Here's how the part is built. I have some questions about the finished solid (model axes, mm). A direction names the side the tool comes from. Round coordinates to 2 decimals unless told otherwise and drop trailing zeros. Loops run counter-clockwise (first coordinate to the right, second up) from the corner with the lowest first, then second, coordinate; pieces in that order, holes last. Notation, with made-up numbers: (59, -9) -> (95, -9) arc R22 cw to (95, -3) -> close; hole circle Ø8 at (60, 60). An arc over 180 degrees is marked (long way). One line per item, written item: value. Start each with the question number.
```python
from build123d import *

# Parameters (mm, degrees)
AUFSATZ_LINEAR_AUSTRAGEN1_OUTLINE_W = 29
AUFSATZ_LINEAR_AUSTRAGEN1_OUTLINE_H = 29
AUFSATZ_LINEAR_AUSTRAGEN1_DEPTH     = 2
SKIZZE2_W                           = 19
SKIZZE2_H                           = 24
AUFSATZ_LINEAR_AUSTRAGEN2_DEPTH     = 18
SKIZZE5_W                           = 15
SKIZZE5_H                           = 24
SCHNITT_LINEAR_AUSTRAGEN2_DEPTH     = 15
SCHNITT_LINEAR_AUSTRAGEN3_REACH     = 44.626
SKIZZE4_R                           = 1.25
SKIZZE6_W                           = 35
SKIZZE6_H                           = 24
AUFSATZ_LINEAR_AUSTRAGEN3_DEPTH     = 7
SKIZZE9_R                           = 2
SCHNITT_LINEAR_AUSTRAGEN4_DEPTH     = 5
SKIZZE19_W                          = 17
SKIZZE19_H                          = 5
SCHNITT_LINEAR_AUSTRAGEN15_DEPTH    = 2
SKIZZE20_R                          = 1.5
SCHNITT_LINEAR_AUSTRAGEN16_DEPTH    = 2
SKIZZE21_W                          = 7
SKIZZE21_H                          = 8
SCHNITT_LINEAR_AUSTRAGEN17_DEPTH    = 2
SKIZZE23_W                          = 6.5
SKIZZE23_H                          = 5
SKIZZE23_W_2                        = 5.5
SCHNITT_LINEAR_AUSTRAGEN18_DEPTH    = 2
SKIZZE24_W                          = 29
SKIZZE24_H                          = 2
AUFSATZ_LINEAR_AUSTRAGEN4_DEPTH     = 5
SKIZZE25_R                          = 1
SCHNITT_LINEAR_AUSTRAGEN19_DEPTH    = 2
SKIZZE26_W                          = 35
SKIZZE26_H                          = 3
SCHNITT_LINEAR_AUSTRAGEN20_DEPTH    = 7
SKIZZE27_R                          = 3.5
SCHNITT_LINEAR_AUSTRAGEN21_DEPTH    = 2


# Read off the part's stored shape, not the designer's step: Aufsatz-Linear austragen1
with BuildPart() as part:
    # Aufsatz-Linear austragen1 outline → Aufsatz-Linear austragen1 (new body)
    with BuildSketch(Plane.XY):
        with Locations((14.5, 14.5)):
            Rectangle(AUFSATZ_LINEAR_AUSTRAGEN1_OUTLINE_W, AUFSATZ_LINEAR_AUSTRAGEN1_OUTLINE_H)
    extrude(amount=AUFSATZ_LINEAR_AUSTRAGEN1_DEPTH)

    # Skizze2 → Aufsatz-Linear austragen2 (add)
    with BuildSketch(Plane.XY.offset(2)):
        with Locations((14.5, 17)):
            Rectangle(SKIZZE2_W, SKIZZE2_H)
    extrude(amount=AUFSATZ_LINEAR_AUSTRAGEN2_DEPTH)

    # Skizze5 → Schnitt-Linear austragen2 (cut)
    with BuildSketch(Plane.XY.offset(20)):
        with Locations((14.5, 17)):
            Rectangle(SKIZZE5_W, SKIZZE5_H)
    extrude(amount=-SCHNITT_LINEAR_AUSTRAGEN2_DEPTH, mode=Mode.SUBTRACT)

    # Schnitt-Linear austragen3: up to this face of the body (flat: up to its plane)
    schnitt_linear_austragen3_end = Plane(part.part.faces().sort_by_distance((24, 17, 11))[0])
    # Skizze4 → Schnitt-Linear austragen3 (cut, up to the picked face)
    with BuildSketch(Plane.ZY.offset(-5), mode=Mode.PRIVATE) as schnitt_linear_austragen3_sk1:
        with Locations((12, 15)):
            Circle(SKIZZE4_R)
    schnitt_linear_austragen3_tool1 = split(extrude(schnitt_linear_austragen3_sk1.sketch, amount=-SCHNITT_LINEAR_AUSTRAGEN3_REACH, mode=Mode.PRIVATE), bisect_by=schnitt_linear_austragen3_end, keep=Keep.BOTH, mode=Mode.PRIVATE)
    add(schnitt_linear_austragen3_tool1.solids().sort_by(Axis((5, 15, 12), (1, 0, 0)))[0], mode=Mode.SUBTRACT)

    # Skizze6 → Aufsatz-Linear austragen3 (add)
    with BuildSketch(Plane.XY.offset(20)):
        with Locations((14.5, 17)):
            Rectangle(SKIZZE6_W, SKIZZE6_H)
    extrude(amount=AUFSATZ_LINEAR_AUSTRAGEN3_DEPTH)

    # Skizze9 → Schnitt-Linear austragen4 (cut)
    with BuildSketch(Plane(origin=(0, 0, 20), x_dir=(-1, 0, 0), z_dir=(0, 0, -1))):
        with Locations((-1.5, 14)):
            Circle(SKIZZE9_R)
        with Locations((-27.5, 14)):
            Circle(SKIZZE9_R)
    extrude(amount=-SCHNITT_LINEAR_AUSTRAGEN4_DEPTH, mode=Mode.SUBTRACT)

    # Skizze19 → Schnitt-Linear austragen15 (cut)
    with BuildSketch(Plane(origin=(0, 0, 0), x_dir=(-1, 0, 0), z_dir=(0, 0, -1))):
        with Locations((-14, 2.5)):
            Rectangle(SKIZZE19_W, SKIZZE19_H)
    extrude(amount=-SCHNITT_LINEAR_AUSTRAGEN15_DEPTH, mode=Mode.SUBTRACT)

    # Skizze20 → Schnitt-Linear austragen16 (cut)
    with BuildSketch(Plane(origin=(0, 0, 25), x_dir=(-1, 0, 0), z_dir=(0, 0, -1))):
        with Locations((-27.5, 14)):
            Circle(SKIZZE20_R)
        with Locations((-1.5, 14)):
            Circle(SKIZZE20_R)
    extrude(amount=-SCHNITT_LINEAR_AUSTRAGEN16_DEPTH, mode=Mode.SUBTRACT)

    # Skizze21 → Schnitt-Linear austragen17 (cut)
    with BuildSketch(Plane.XY.offset(5)):
        with Locations((14.5, 25)):
            Rectangle(SKIZZE21_W, SKIZZE21_H)
    extrude(amount=-SCHNITT_LINEAR_AUSTRAGEN17_DEPTH, mode=Mode.SUBTRACT)

    # Skizze23 → Schnitt-Linear austragen18 (cut)
    with BuildSketch(Plane(origin=(0, 0, 0), x_dir=(-1, 0, 0), z_dir=(0, 0, -1))):
        with Locations((-25.75, 2.5)):
            Rectangle(SKIZZE23_W, SKIZZE23_H)
        with Locations((-2.75, 2.5)):
            Rectangle(SKIZZE23_W_2, SKIZZE23_H)
    extrude(amount=-SCHNITT_LINEAR_AUSTRAGEN18_DEPTH, mode=Mode.SUBTRACT)

    # Skizze24 → Aufsatz-Linear austragen4 (add)
    with BuildSketch(Plane(origin=(0, 29, 0), x_dir=(1, 0, 0), z_dir=(0, 1, 0))):
        with Locations((14.5, -1)):
            Rectangle(SKIZZE24_W, SKIZZE24_H)
    extrude(amount=AUFSATZ_LINEAR_AUSTRAGEN4_DEPTH)

    # Skizze25 → Schnitt-Linear austragen19 (cut)
    with BuildSketch(Plane(origin=(0, 0, 0), x_dir=(-1, 0, 0), z_dir=(0, 0, -1))):
        with Locations((-1.75, 32.25)):
            Circle(SKIZZE25_R)
        with Locations((-27.25, 32.25)):
            Circle(SKIZZE25_R)
        with Locations((-27.25, 6.75)):
            Circle(SKIZZE25_R)
        with Locations((-1.75, 6.75)):
            Circle(SKIZZE25_R)
    extrude(amount=-SCHNITT_LINEAR_AUSTRAGEN19_DEPTH, mode=Mode.SUBTRACT)

    # Skizze26 → Schnitt-Linear austragen20 (cut)
    with BuildSketch(Plane.XY.offset(27)):
        with Locations((14.5, 27.5)):
            Rectangle(SKIZZE26_W, SKIZZE26_H)
    extrude(amount=-SCHNITT_LINEAR_AUSTRAGEN20_DEPTH, mode=Mode.SUBTRACT)

    # Skizze27 → Schnitt-Linear austragen21 (cut)
    with BuildSketch(Plane(origin=(0, 0, 0), x_dir=(-1, 0, 0), z_dir=(0, 0, -1))):
        with Locations((-27.5, 14)):
            Circle(SKIZZE27_R)
        with Locations((-1.5, 14)):
            Circle(SKIZZE27_R)
    extrude(amount=-SCHNITT_LINEAR_AUSTRAGEN21_DEPTH, mode=Mode.SUBTRACT)


solid = part.part
```
Q1. Will these pins go through, and if not, where does the flat tip stop? P1, Ø0.6, axis at x = 16, z = 4.5, coming from the +Y side; P2, Ø5, axis at y = 14, z = 17, coming from the -X side; P3, Ø1, axis at y = 24.5, z = 4, coming from the +X side.
Q2. If we mould it in two halves opening along Z, with no side actions, what happens to faces 5 (the flat face through (23, 28, 20)), 6 (the flat face through (14, 26, 24)), 7 (the flat face through (11, 31, 2))? For each: released by +Z, released by -Z, zero draft, split by the parting line, or undercut.
Q3. I want a section at A-A on y = 32.25. Please give me the cut outline in (x, z), plus the area to 3 significant figures.
Q4. I want a section at C-C on z = 18.75. Please give me the cut outline in (x, y), plus the area to 3 significant figures.
Q5. I want a section at B-B on x = 12. Please give me the cut outline in (y, z), plus the area to 3 significant figures.
Q6. I want a section at D-D on y = 6.75. Please give me the cut outline in (x, z), plus the area to 3 significant figures.
Q7. If I drill on line 1 along Y through (x, z) = (27.5, 22.3); line 2 along Z through (x, y) = (8, 23.25); line 3 along X through (y, z) = (28.5, 17), over which ranges is the centre line in solid material (lowest first)?
Q8. Which directions (+Z, -Z, +X, -X, +Y, -Y) give clear straight access to the entire face, cutting with the end or side of a thin tool? Please do faces 1 (the flat face through (29, 8, 1)), 2 (the flat face through (18, 25, 4)), 3 (the flat face through (0, 25, 1)), 4 (the cylindrical face through (27.987, 7.426, 0.986)).
Answers below:
1. P1: stops at y = 21
1. P2: stops at x = 5
1. P3: stops at x = 24
2. face 5: released by +Z
2. face 6: zero draft
2. face 7: undercut
3. outline: (0, 0) -> (0.75, 0) -> (0.75, 2) -> (0, 2) -> close; (2.75, 0) -> (26.25, 0) -> (26.25, 2) -> (2.75, 2) -> close; (28.25, 0) -> (29, 0) -> (29, 2) -> (28.25, 2) -> close
3. area: 50.0 mm^2
4. outline: (5, 5) -> (7, 5) -> (7, 29) -> (5, 29) -> close; (22, 5) -> (24, 5) -> (24, 29) -> (22, 29) -> close
4. area: 96.0 mm^2
5. outline: (5, 0) -> (34, 0) -> (34, 2) -> (29, 2) -> (29, 3) -> (21, 3) -> (21, 5) -> (5, 5) -> close; (5, 20) -> (26, 20) -> (26, 27) -> (5, 27) -> close
5. area: 261 mm^2
6. outline: (-3, 20) -> (5, 20) -> (5, 2) -> (2.75, 2) -> (2.75, 0) -> (26.25, 0) -> (26.25, 2) -> (24, 2) -> (24, 20) -> (32, 20) -> (32, 27) -> (-3, 27) -> close; (0, 0) -> (0.75, 0) -> (0.75, 2) -> (0, 2) -> close; (28.25, 0) -> (29, 0) -> (29, 2) -> (28.25, 2) -> close; hole (7, 5) -> (22, 5) -> (22, 20) -> (7, 20) -> close
6. area: 412 mm^2
7. line 1: y = 5 to 12, 16 to 26
7. line 2: z = 0 to 5, 20 to 27
7. line 3: x = 5 to 7, 22 to 24
8. face 1: -Z, +X, +Y, -Y
8. face 2: +Y
8. face 3: -Z, -X, +Y, -Y
8. face 4: -Z
